Part print with two shaded views. Sizes in mm from the minimum x, y, z corner. Round coordinates to 2 decimals unless told otherwise and drop trailing zeros. Loops run counter-clockwise (first coordinate to the right, second up) from the corner with the lowest first, then second, coordinate; pieces in that order, holes last. Notation, with made-up numbers: M 4,43.25 L 38,43.25 A33 ccw 38,74.25 Z; hole C 70.5,83.5 d9. An arc over 180 degrees is marked long. Answer as CSV lines item,"result". Start each with the question number.
Item 1: Band-saw the part on A-A (z = 4). Give the cut face in (x, y), and give its area (3 significant figures).
Item 2: Drop a flat-ended pin along its axis: pin 1 Ø3.5 at (x, z) = (4, 4) entering from -Y. Give the stop position or say it passes through.
Item 3: Mould opens along X. For the marked faces 1, 2 and 3 say: pulls with the +X half, pulls with the -X half, needs draft (parallel to the pull), parting line crosses it, or undercut.
Item 4: Band-saw the part on C-C (y = 0.4). Give the cut face in (x, z).
Item 5: Wall check: line 1 (Z direction, x = 4, y = 3); line 2 (X direction, y = 0.4, z = 3.5); line 3 (Z direction, x = 4.75, y = 1.6). Give the ranges that are in metal, low to high.
Item 6: Band-saw the part on B-B (x = 4). Give the cut face in (y, z), and give its area (3 significant figures).
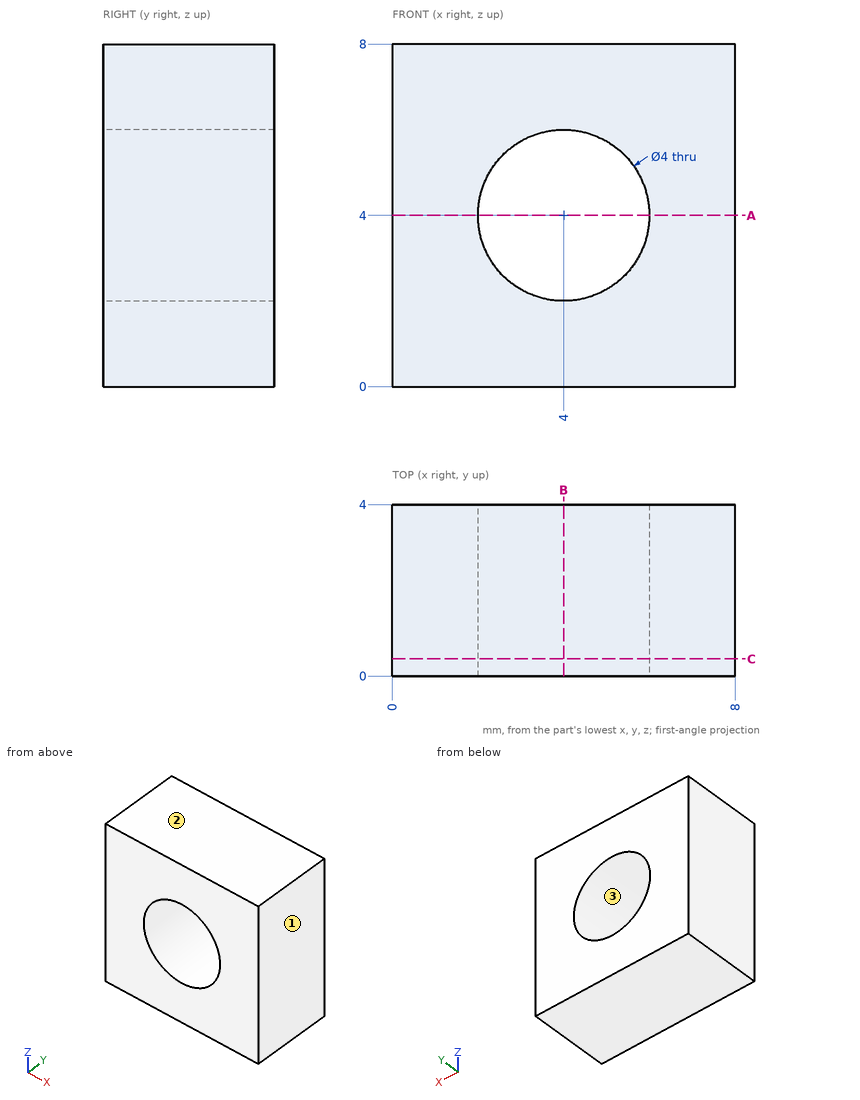
Answer block:
1,outline,"M 0,0 L 2,0 L 2,4 L 0,4 Z; M 6,0 L 8,0 L 8,4 L 6,4 Z"
1,area,"16.0 mm^2"
2,pin 1,"passes through"
3,face 1,"pulls with the +X half"
3,face 2,"needs draft"
3,face 3,"undercut"
4,outline,"M 0,0 L 8,0 L 8,8 L 0,8 Z; hole C 4,4 d4"
5,line 1,"z = 0 to 2, 6 to 8"
5,line 2,"x = 0 to 2.06, 5.94 to 8"
5,line 3,"z = 0 to 2.15, 5.85 to 8"
6,outline,"M 0,0 L 4,0 L 4,2 L 0,2 Z; M 0,6 L 4,6 L 4,8 L 0,8 Z"
6,area,"16.0 mm^2"
